Part model, mm, in its own coordinate system. A direction names the side the tool comes from. Give positions to 0.01 mm unless a question says otherwise; leave off trailing zeros. Write each loop counter-clockwise with the first axis right and the second up, starting at its lowest first coordinate (ties: lowest second). Pieces come first, ordered by that corner, then holes. Notation, with made-up numbers: M 84.5,-18 L 113.5,-18 A23 cw 113.5,-5 Z; hole C 87.5,-1.75 d2. An arc over 180 degrees is marked long. Answer as CSV lines item,"result". Start each with the question number.
1) Slice it at B-B, the plane y = -35. Give the cut face in (x, z), plus the area to 3 significant figures.
2) Slice it at A-A, the plane y = -19. Give the cut face in (x, z).
3) Slice it at D-D, the plane x = 295. Give the cut face in (y, z), plus the area to 3 significant figures.
4) Pin check, flat tips, straight feed: pin 1 Ø10 at (y, z) = (-8, 156.5) entering from +X; pin 2 Ø4 at (y, z) = (-29.5, 197.5) entering from +X; pin 3 Ø11 at (x, z) = (162, 155.5) entering from +Y; pin 4 Ø12 at (x, z) = (246.5, 225.5) entering from +Y. Stop position of each tip, or through.
5) Slice it at C-C, the plane z = 146. Give the cut face in (x, y).
6) Tool access for faces 1 (the flat face through (170, -25.4, 153)), 2 (the flat face through (211, 0, 196)): list every direction of +Z, -Z, +X, -X, +Y, -Y with a clear straight run to the whole face (end or side of a thin tool).
7) Wall check: line 1 along X through (y, z) = (-7, 199); line 2 along X through (y, z) = (-26.5, 232); line 3 along Z through (x, y) = (115.5, -38). Give the ranges that are in metal, low to high. Write a range as from..to.
```python
from build123d import *

# Parameters (mm, degrees)
F1_DEPTH = 50.8
F3_DEPTH = 25.4


with BuildPart() as f1:
    # F0 (on Front) → F1 (new body)
    with BuildSketch(Plane.XZ):
        Polygon((304.807853, 304.807853), (0, 0), (35.921024, 0), (318.142853, 282.221829), (318.142853, 304.807853), align=None)
    extrude(amount=F1_DEPTH)

    # F2 (on Front) → F3 (cut)
    with BuildSketch(Plane.XZ):
        Polygon((235.138051, 267.217477), (217.177538, 249.256964), (266.149292, 200.285211), (284.109804, 218.245724), align=None)
        Polygon((77.603452, 101.462855), (59.64294, 83.502342), (106.885168, 36.260115), (124.84568, 54.220627), align=None)
        Polygon((151.667562, 189.043356), (133.707049, 171.082843), (190.513352, 114.27654), (208.473865, 132.237053), align=None)
    extrude(amount=F3_DEPTH, mode=Mode.SUBTRACT)


solid = f1.part
```
Found:
1,outline,"M 0,0 L 35.92,0 L 318.14,282.22 L 318.14,304.81 L 304.81,304.81 Z"
1,area,"10,700 mm²"
2,outline,"M 0,0 L 35.92,0 L 89.53,53.61 L 71.57,71.57 Z; M 89.53,89.53 L 107.49,71.57 L 170.36,134.43 L 152.39,152.39 Z; M 170.36,170.36 L 188.32,152.39 L 251.18,215.26 L 233.22,233.22 Z; M 251.18,251.18 L 269.14,233.22 L 318.14,282.22 L 318.14,304.81 L 304.81,304.81 Z"
3,outline,"M -50.8,259.08 L 0,259.08 L 0,295 L -50.8,295 Z"
3,area,"1,820 mm²"
4,pin 1,"x = 197.42"
4,pin 2,"x = 235.42"
4,pin 3,"y = -25.4"
4,pin 4,"y = 0"
5,outline,"M 146,-50.8 L 181.92,-50.8 L 181.92,-25.4 L 158.79,-25.4 L 158.79,0 L 146,0 Z"
6,face 1,"+Y"
6,face 2,"+Z, -Z, +X, -X, +Y"
7,line 1,"199..234.92"
7,line 2,"232..267.92"
7,line 3,"79.58..115.5"
